Design review of the part built by this model. Coordinates are the model's own, in mm. A direction names the side the tool comes from. Coordinates: 2 decimals unless noted, no trailing zeros. Order: outer loops, then holes, each group sorted by start corner. A loop starts at its lowest first (then second) coordinate and runs counter-clockwise, first axis right, second up. Notation, with made-up numbers: M -21.75,86 L 26.25,86 A14 ccw 26.25,112 Z; hole C -40,73.25 d7. An arc over 180 degrees is marked long. Use CSV: the item, a comma, the result in double quotes.
```python
from build123d import *

# Parameters (mm, degrees)
SKETCH2_R           = 35.85
BOSS_EXTRUDE3_DEPTH = 11.802411407
SKETCH3_R           = 13.25
CUT_EXTRUDE1_DEPTH  = 6
SHELL1_T            = -10
CUT_EXTRUDE2_START  = -6
SKETCH4_R           = 23.25
CUT_EXTRUDE2_DEPTH  = 6
CUT_EXTRUDE3_START  = -4
SKETCH5_R           = 25.85
CUT_EXTRUDE3_DEPTH  = 4
SKETCH6_R           = 2.4
CUT_EXTRUDE4_DEPTH  = 18
BOSS_EXTRUDE4_START = 2
SKETCH7_R           = 35.85
BOSS_EXTRUDE4_DEPTH = 2
SKETCH8_R           = 5
SKETCH8_R_2         = 13.25
CUT_EXTRUDE6_DEPTH  = 2


with BuildPart() as part:
    # Sketch2 → Boss-Extrude3 (new body)
    with BuildSketch(Plane(origin=(0, 0, 0), x_dir=(1, 0, 0), z_dir=(0, 1, 0))):
        with Locations(Location((0, 0, 0), (0, 0, 270))):
            Circle(SKETCH2_R)
    extrude(amount=BOSS_EXTRUDE3_DEPTH)

    # Sketch3 → Cut-Extrude1 (cut)
    with BuildSketch(Plane.XZ):
        with Locations(Location((0, 0, 0), (0, 0, 270))):
            Circle(SKETCH3_R)
    extrude(amount=-CUT_EXTRUDE1_DEPTH, mode=Mode.SUBTRACT)

    # Shell1
    shell1_openings = [part.faces().sort_by_distance(p)[0] for p in [
        (0, 11.802411407, 0),
    ]]
    offset(amount=SHELL1_T, openings=shell1_openings, kind=Kind.INTERSECTION)

    # Sketch4 → Cut-Extrude2 (cut)
    with BuildSketch(Plane(origin=(0, 16, 0), x_dir=(1, 0, 0), z_dir=(0, 1, 0)).offset(CUT_EXTRUDE2_START)):
        Circle(SKETCH4_R)
    extrude(amount=CUT_EXTRUDE2_DEPTH, mode=Mode.SUBTRACT)

    # Sketch5 → Cut-Extrude3 (cut)
    with BuildSketch(Plane(origin=(0, 10, 0), x_dir=(1, 0, 0), z_dir=(0, 1, 0)).offset(CUT_EXTRUDE3_START)):
        with Locations(Location((0, 0, 0), (0, 0, 270))):
            Circle(SKETCH5_R)
    extrude(amount=CUT_EXTRUDE3_DEPTH, mode=Mode.SUBTRACT)

    # Sketch6 → Cut-Extrude4 (cut)
    with BuildSketch(Plane.XZ):
        with Locations(Location((-19.408408583, -6.6002785, 0), (0, 0, 270))):
            Circle(SKETCH6_R)
        with Locations(Location((19.408408583, 6.6002785, 0), (0, 0, 270))):
            Circle(SKETCH6_R)
    extrude(amount=-CUT_EXTRUDE4_DEPTH, mode=Mode.SUBTRACT)

    # Sketch7 → Boss-Extrude4 (add)
    with BuildSketch(Plane.XZ.offset(BOSS_EXTRUDE4_START)):
        with Locations(Location((0, 0, 0), (0, 0, 270))):
            Circle(SKETCH7_R)
    extrude(amount=-BOSS_EXTRUDE4_DEPTH)

    # Sketch8 → Cut-Extrude6 (cut)
    with BuildSketch(Plane.XZ.offset(2)):
        with Locations(Location((-19.408408583, -6.6002785, 0), (0, 0, 270))):
            Circle(SKETCH8_R)
        with Locations(Location((19.408408583, 6.6002785, 0), (0, 0, 270))):
            Circle(SKETCH8_R)
        with Locations(Location((0, 0, 0), (0, 0, 270))):
            Circle(SKETCH8_R_2)
    extrude(amount=-CUT_EXTRUDE6_DEPTH, mode=Mode.SUBTRACT)


solid = part.part
```
(1) Add section A-A on x = 0. State the section outline as (y, z) points.
The answers:
outline,"M -2,-35.85 L 11.8,-35.85 L 11.8,-25.85 L 6,-25.85 L 6,-13.25 L -2,-13.25 Z; M -2,13.25 L 6,13.25 L 6,25.85 L 11.8,25.85 L 11.8,35.85 L -2,35.85 Z"
(2) Add section C-C on y = 7. State the section outline as (x, z) points.
The answers:
outline,"C 0,0 d71.7; hole C 0,0 d51.7"
(3) The part is to be moulded in two halves that separate along Z. For faces 4 (the face through (6, 6, -12)), 5 (the face through (11, 11.802, 24)), say which applies: pulls with the +Z half, pulls with the -Z half, needs draft (parallel to the pull), parting line crosses it, or undercut.
The answers:
face 4,"undercut"
face 5,"needs draft"
(4) Clearance check with flat-ended pins moving along their axes: P1, Ø1, axis at x = -15.5, y = -0.5, coming from the +Z side; P2, Ø3, axis at y = 3, z = 11.5, coming from the -X side; P3, Ø3, axis at x = -19.41, z = -6.6, coming from the +Y side; P4, Ø3, axis at x = 14.5, y = 4.5, coming from the +Z side. State where each tip first meets the part, or that it passes through.
The answers:
P1,"stops at z = 32.56"
P2,"stops at x = -34.43"
P3,"passes through"
P4,"stops at z = 33.41"
(5) Add section D-D on z = -21.5. State the section outline as (x, y) points.
The answers:
outline,"M -28.69,-2 L 28.69,-2 L 28.69,11.8 L 14.35,11.8 L 14.35,6 L -14.35,6 L -14.35,11.8 L -28.69,11.8 Z"
(6) For faces 1 (the face through (1, -2, -15)), 2 (the face through (-18, 0, -9)), 3 (the face through (-15.729, 8.861, -20.514)), list the 3-axis set-ups (+Z, -Z, +X, -X, +Y, -Y) from which the entire face can be reached by the end or side of a thin tool; tool diameter is ignored.
The answers:
face 1,"+Z, -Z, +X, -X, -Y"
face 2,"-Y"
face 3,"+Y"
(7) Add section B-B on z = 0. State the section outline as (x, y) points, and give its area (3 significant figures).
The answers:
outline,"M -35.85,-2 L -13.25,-2 L -13.25,6 L -25.85,6 L -25.85,11.8 L -35.85,11.8 Z; M 13.25,-2 L 35.85,-2 L 35.85,11.8 L 25.85,11.8 L 25.85,6 L 13.25,6 Z"
area,"478 mm2"
(8) Wall thickness on probe 1 along X at (y, z) = (-0.5, -2); probe 2 along X at (y, z) = (3, -8.5); probe 3 along X at (y, z) = (-0.75, 0): over which ranges is each line inside the solid? List them lowest first.
The answers:
probe 1,"x = -35.79 to -21.37, -17.45 to -13.1, 13.1 to 35.79"
probe 2,"x = -34.83 to -20.88, -17.94 to -10.16, 10.16 to 34.83"
probe 3,"x = -35.85 to -13.25, 13.25 to 35.85"
